from build123d import *

# Parameters (mm, degrees)
F0_W     = 8.89
F0_H     = 8.89
F1_DEPTH = 40.64
F2_W     = 8.89
F2_H     = 34.29
F3_DEPTH = 8.89
F4_R     = 2.54


with BuildPart() as f1:
    # F0 (on Front) → F1 (new body)
    with BuildSketch(Plane.XZ):
        with Locations((0.729244, 0.33937)):
            Rectangle(F0_W, F0_H)
    extrude(amount=F1_DEPTH)

    # F2 (on face) → F3 (join)
    with BuildSketch(Plane.XZ.offset(40.64)):
        with Locations((0.729244, 13.03937)):
            Rectangle(F2_W, F2_H)
    extrude(amount=F3_DEPTH)

    # F4
    f4_edges = [f1.edges().sort_by_distance(p)[0] for p in [
        (5.174244, -40.64, 17.48437),
        (0.729244, -40.64, 30.18437),
        (-3.715756, -40.64, 17.48437),
        (-3.715756, -45.085, 30.18437),
        (-3.715756, -49.53, 13.03937),
        (-3.715756, -20.32, 4.78437),
        (-3.715756, -24.765, -4.10563),
        (5.174244, -20.32, 4.78437),
        (5.174244, -49.53, 13.03937),
        (5.174244, -24.765, -4.10563),
        (0.729244, -49.53, -4.10563),
        (5.174244, -45.085, 30.18437),
        (0.729244, -49.53, 30.18437),
    ]]
    fillet(f4_edges, radius=F4_R)


solid = f1.part
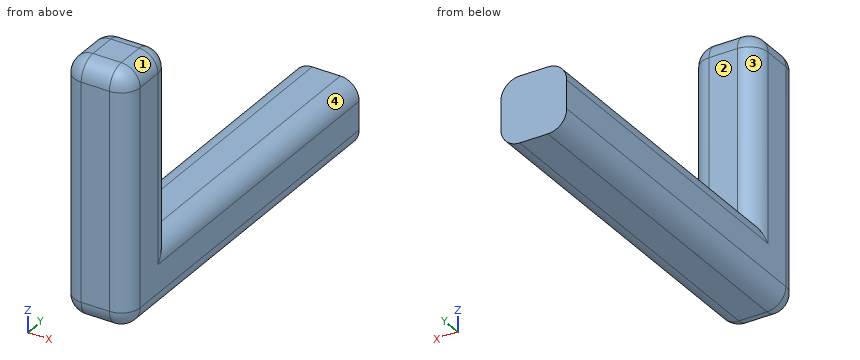
Model file for the job. Use its own axes, mm. Face numbers are marked on the shaded views. A direction names the side the tool comes from. Round coordinates to 2 decimals unless told otherwise and drop trailing zeros. Order: outer loops, then holes, each group sorted by start corner. A loop starts at its lowest first (then second) coordinate and runs counter-clockwise, first axis right, second up. Notation, with made-up numbers: M -19,19.5 L -1,19.5 A10 cw -1,37.5 Z; hole C -27.75,-12.5 d7. An arc over 180 degrees is marked long. Write each question's results on one line, items separated by ' | '. Start each with the question number.
(1) Saw through at D-D, the plane z = 3. Give the cut face in (x, y).
(2) Probe probe 1 along Z at (x, y) = (1.75, -32.5); probe 2 along Y at (x, z) = (2.5, 19.5); probe 3 along Y at (x, z) = (3.75, 5.5). List the from-to ranges inside material, lowest first. Write a range as from..to.
(3) Saw through at B-B, the plane x = 0.75. Give the cut face in (y, z).
(4) Saw through at A-A, the plane z = 9. Give the cut face in (x, y), then the cut area to 3 significant figures.
(5) Which spindle directions (+Z, -Z, +X, -X, +Y, -Y) get a long thin tool onto all of the face, cutting with end or side? Do the marked faces 1, 2, 3 and 4. Say none if no direction does.
(6) Saw through at C-C, the plane y = -4. Give the cut face in (x, z).
(7) Drop flat-ended pins along their axis: pin 1 (3 mm diameter, centred on x = -0.5, z = 18, fed in from +Y); pin 2 (1.9 mm diameter, centred on x = 1, y = -15.5, fed in from +Z); pin 3 (10 mm diameter, centred on y = -34.5, z = 23.5, fed in from +X) (3 decimals). Give the stop position or say it passes through.
Established:
1) outline: M -3.72,-46.99 A2.54 ccw -1.18,-49.53 L 2.63,-49.53 A2.54 ccw 5.17,-46.99 L 5.17,-43.18 A2.54 ccw 5.06,-42.42 L 5.06,0 L -3.6,0 L -3.6,-42.42 A2.54 ccw -3.72,-43.18 Z
2) probe 1: z = -4.11..4.78 | probe 2: y = -49.53..-40.64 | probe 3: y = -49.27..-40.9
3) outline: M -49.53,-1.57 A2.54 ccw -46.99,-4.11 L 0,-4.11 L 0,4.78 L -40.64,4.78 L -40.64,27.64 A2.54 ccw -43.18,30.18 L -46.99,30.18 A2.54 ccw -49.53,27.64 Z
4) outline: M -3.72,-46.99 A2.54 ccw -1.18,-49.53 L 2.63,-49.53 A2.54 ccw 5.17,-46.99 L 5.17,-43.18 A2.54 ccw 2.63,-40.64 L -1.18,-40.64 A2.54 ccw -3.72,-43.18 Z | area: 73.5 mm^2
5) face 1: +Z, +X, +Y, -Y | face 2: +Z, +X, -X, +Y | face 3: +Z, -X, +Y | face 4: +Z, +X, +Y
6) outline: M -3.72,-1.57 A2.54 ccw -1.18,-4.11 L 2.63,-4.11 A2.54 ccw 5.17,-1.57 L 5.17,2.24 A2.54 ccw 2.63,4.78 L -1.18,4.78 A2.54 ccw -3.72,2.24 Z
7) pin 1: stops at y = -40.64 | pin 2: stops at z = 4.78 | pin 3: passes through
